from build123d import *

# Parameters (mm, degrees)
SKETCH_1_R          = 2.2
EXTRUDE_1_DEPTH     = 5
SKETCH_2_W          = 5
SKETCH_2_H          = 220.282443136
SKETCH_2_H_2        = 219.868690955
CUT_EXTRUDE_1_DEPTH = 10
SKETCH_3_W          = 5
SKETCH_3_H          = 40
EXTRUDE_3_DEPTH     = 5
SKETCH_4_W          = 390.4211829
SKETCH_4_H          = 264.690207343
EXTRUDE_4_DEPTH     = 5
SKETCH_5_R          = 2.2
CUT_EXTRUDE_2_DEPTH = 5
CUT_EXTRUDE_3_DEPTH = 10


with BuildPart() as part:
    # 草图1 → 凸台-拉伸1 (new body)
    with BuildSketch(Plane.XY):
        Polygon((-200, 150), (200, 150), (200, 110), (205, 110), (205, 70), (200, 70), (200, 30), (205, 30), (205, -30), (200, -30), (200, -70), (205, -70), (205, -110), (200, -110), (200, -150), (160, -150), (160, -155), (120, -155), (120, -150), (80, -150), (80, -155), (40, -155), (40, -150), (-40, -150), (-40, -155), (-80, -155), (-80, -150), (-120, -150), (-120, -155), (-160, -155), (-160, -150), (-200, -150), (-200, -110), (-205, -110), (-205, -70), (-200, -70), (-200, -30), (-205, -30), (-205, 30), (-200, 30), (-200, 70), (-205, 70), (-205, 110), (-200, 110), align=None)
        with Locations((-140, -140)):
            Circle(SKETCH_1_R, mode=Mode.SUBTRACT)
        with Locations((-100, -140)):
            Circle(SKETCH_1_R, mode=Mode.SUBTRACT)
        with Locations((-60, -140)):
            Circle(SKETCH_1_R, mode=Mode.SUBTRACT)
        with Locations((-20, -140)):
            Circle(SKETCH_1_R, mode=Mode.SUBTRACT)
        with Locations((20, -140)):
            Circle(SKETCH_1_R, mode=Mode.SUBTRACT)
        with Locations((60, -140)):
            Circle(SKETCH_1_R, mode=Mode.SUBTRACT)
        with Locations((100, -140)):
            Circle(SKETCH_1_R, mode=Mode.SUBTRACT)
        with Locations((140, -140)):
            Circle(SKETCH_1_R, mode=Mode.SUBTRACT)
        with Locations((-190, 110)):
            Circle(SKETCH_1_R, mode=Mode.SUBTRACT)
        with Locations((-190, 70)):
            Circle(SKETCH_1_R, mode=Mode.SUBTRACT)
        with Locations((-190, 30)):
            Circle(SKETCH_1_R, mode=Mode.SUBTRACT)
        with Locations((-190, -30)):
            Circle(SKETCH_1_R, mode=Mode.SUBTRACT)
        with Locations((-190, -70)):
            Circle(SKETCH_1_R, mode=Mode.SUBTRACT)
        with Locations((-190, -110)):
            Circle(SKETCH_1_R, mode=Mode.SUBTRACT)
        with Locations((190, -110)):
            Circle(SKETCH_1_R, mode=Mode.SUBTRACT)
        with Locations((190, -70)):
            Circle(SKETCH_1_R, mode=Mode.SUBTRACT)
        with Locations((190, -30)):
            Circle(SKETCH_1_R, mode=Mode.SUBTRACT)
        with Locations((190, 30)):
            Circle(SKETCH_1_R, mode=Mode.SUBTRACT)
        with Locations((190, 70)):
            Circle(SKETCH_1_R, mode=Mode.SUBTRACT)
        with Locations((190, 110)):
            Circle(SKETCH_1_R, mode=Mode.SUBTRACT)
    extrude(amount=EXTRUDE_1_DEPTH)

    # 草图2 → 切除-拉伸1 (cut)
    with BuildSketch(Plane.XY.offset(5)):
        with Locations((-202.5, -0.141221568)):
            Rectangle(SKETCH_2_W, SKETCH_2_H)
        with Locations((202.5, 0.065654522)):
            Rectangle(SKETCH_2_W, SKETCH_2_H_2)
    extrude(amount=-CUT_EXTRUDE_1_DEPTH, mode=Mode.SUBTRACT)

    # 草图3 → 凸台-拉伸3 (add)
    with BuildSketch(Plane.XY.offset(5)):
        with Locations((-202.5, 130)):
            Rectangle(SKETCH_3_W, SKETCH_3_H)
        with Locations((-202.5, 50)):
            Rectangle(SKETCH_3_W, SKETCH_3_H)
        with Locations((-202.5, -50)):
            Rectangle(SKETCH_3_W, SKETCH_3_H)
        with Locations((-202.5, -130)):
            Rectangle(SKETCH_3_W, SKETCH_3_H)
        with Locations((202.5, -130)):
            Rectangle(SKETCH_3_W, SKETCH_3_H)
        with Locations((202.5, -50)):
            Rectangle(SKETCH_3_W, SKETCH_3_H)
        with Locations((202.5, 50)):
            Rectangle(SKETCH_3_W, SKETCH_3_H)
        with Locations((202.5, 130)):
            Rectangle(SKETCH_3_W, SKETCH_3_H)
    extrude(amount=-EXTRUDE_3_DEPTH)

    # 草图4 → 凸台-拉伸4 (add)
    with BuildSketch(Plane.XY.offset(5)):
        with Locations((1.806920954, 7.46039962)):
            Rectangle(SKETCH_4_W, SKETCH_4_H)
    extrude(amount=-EXTRUDE_4_DEPTH)

    # 草图5 → 切除-拉伸2 (cut)
    with BuildSketch(Plane.XY.offset(5)):
        with Locations((-190, 90)):
            Circle(SKETCH_5_R)
        with Locations((-190, 50)):
            Circle(SKETCH_5_R)
        with Locations((-190, 0)):
            Circle(SKETCH_5_R)
        with Locations((-190, -50)):
            Circle(SKETCH_5_R)
        with Locations((-190, -90)):
            Circle(SKETCH_5_R)
        with Locations(Location((190, -90, 0), (0, 0, 180))):
            Circle(SKETCH_5_R)
        with Locations(Location((190, -50, 0), (0, 0, 180))):
            Circle(SKETCH_5_R)
        with Locations(Location((190, 0, 0), (0, 0, 180))):
            Circle(SKETCH_5_R)
        with Locations(Location((190, 50, 0), (0, 0, 180))):
            Circle(SKETCH_5_R)
        with Locations(Location((190, 90, 0), (0, 0, 180))):
            Circle(SKETCH_5_R)
    extrude(amount=-CUT_EXTRUDE_2_DEPTH, mode=Mode.SUBTRACT)

    # 草图6 → 切除-拉伸3 (cut)
    with BuildSketch(Plane.XY.offset(5)):
        with BuildLine():
            Line((-60, 50), (60, 50))
            ThreePointArc((60, 50), (80, 30), (60, 10))
            Line((60, 10), (-60, 10))
            ThreePointArc((-60, 10), (-80, 30), (-60, 50))
        make_face()
        with BuildLine():
            Line((-60, 110), (60, 110))
            ThreePointArc((60, 110), (80, 90), (60, 70))
            Line((60, 70), (-60, 70))
            ThreePointArc((-60, 70), (-80, 90), (-60, 110))
        make_face()
    extrude(amount=-CUT_EXTRUDE_3_DEPTH, mode=Mode.SUBTRACT)


solid = part.part
The listing builds one solid part. Answer for the finished solid, in the listing's coordinates (mm). A direction names the side the tool comes from. Coordinates: 2 decimals unless noted, no trailing zeros. Write each loop counter-clockwise with the first axis right and the second up, starting at its lowest first coordinate (ties: lowest second). Pieces come first, ordered by that corner, then holes. Notation, with made-up numbers: (53, 58.5) - (92, 58.5) arc R3 cw to (92, 62.5) - close; hole circle Ø10 at (-3, 13.25). An arc over 180 degrees is marked (long way). Answer as CSV lines item,"result".
1. Find section D-D (x = -110.5). Give the vertices of the cut face in (y, z).
Computed values:
outline,"(-150, 0) - (150, 0) - (150, 5) - (-150, 5) - close"
2. A tool of negligible diameter and unlimited length cuts with its end or side. For faces 3 (the cylindrical face through (-80, 90, 3)), 4 (the flat face through (-3, 0, 5)), from which of +Z, -Z, +X, -X, +Y, -Y can it reach the whole face along a straight path? Write none if from no direction.
Computed values:
face 3,"+Z, -Z"
face 4,"+Z, +X, -X, +Y, -Y"
3. Straight lines are drawn through the part: line 1 (Y direction, x = -100, z = 1.45); line 2 (Y direction, x = -71, z = 2.4); line 3 (Y direction, x = 140, z = 2.85). For each, find the intervals that lie inside material, in ascending order. Write a range as [from, to].
Computed values:
line 1,"y = [-150, -142.2], [-137.8, 150]"
line 2,"y = [-155, 13.3], [46.7, 73.3], [106.7, 150]"
line 3,"y = [-155, -142.2], [-137.8, 150]"
4. Determine the mould class of faces 1 (the cylindrical face through (80, 30, 3)), 2 (the flat face through (-3, 0, 0)) for opening direction X: +X half, -X half, draft (parallel to the pull), parting line (faces both ways), or undercut.
Computed values:
face 1,"undercut"
face 2,"draft"
5. Given P1, Ø2.5, axis at y = -151.5, z = 2.5, coming from the +X side; P2, Ø2.5, axis at x = -20, y = -140, coming from the -Z side; P3, Ø1.5, axis at y = -96, z = 3, coming from the +X side; P4, Ø2.5, axis at y = -151.5, z = 3.5, coming from the -X side, each flat-ended and moving along its own axis, determine where each tip first touches the part or whether it passes through.
Computed values:
P1,"stops at x = 160"
P2,"passes through"
P3,"stops at x = 200"
P4,"stops at x = -160"
6. Find section C-C (y = 22). Give the vertices of the cut face in (x, z), plus the area to 3 significant figures.
Computed values:
outline,"(-200, 0) - (-78.33, 0) - (-78.33, 5) - (-200, 5) - close; (78.33, 0) - (200, 0) - (200, 5) - (78.33, 5) - close"
area,"1,220 mm²"
7. Find section A-A (y = 77). Give the vertices of the cut face in (x, z).
Computed values:
outline,"(-200, 0) - (-75.2, 0) - (-75.2, 5) - (-200, 5) - close; (75.2, 0) - (200, 0) - (200, 5) - (75.2, 5) - close"
8. Find section B-B (z = 2.95). Give the number of separate pieces and of enclosed holes in the cut face, plus the area to 3 significant figures.
Computed values:
separate pieces,"1"
enclosed holes,"20"
area,"110,000 mm²"
